The listing builds one solid part. Answer for the finished solid, in the listing's coordinates (mm). Face numbers are marked on the shaded views. A direction names the side the tool comes from. Coordinates: 2 decimals unless noted, no trailing zeros. Order: outer loops, then holes, each group sorted by start corner. A loop starts at its lowest first (then second) coordinate and runs counter-clockwise, first axis right, second up.
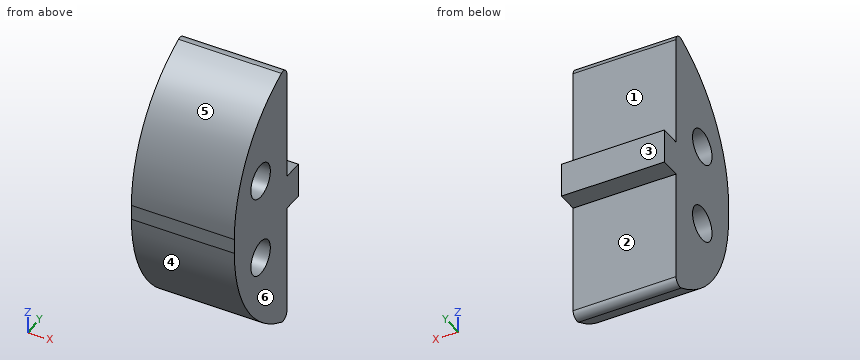
from build123d import *

# Parameters (mm, degrees)
SKETCH1_W           = 30
SKETCH1_H           = 80
BOSS_EXTRUDE1_DEPTH = 27
SKETCH5_W           = 30
SKETCH5_H           = 10
BOSS_EXTRUDE2_DEPTH = 6
SKETCH2_R           = 5
CUT_EXTRUDE1_DEPTH  = 40
FILLET5_R           = 40
FILLET6_R           = 40
FILLET7_R           = 2
FILLET8_R           = 2


with BuildPart() as part:
    # Sketch1 → Boss-Extrude1 (new body)
    with BuildSketch(Plane(origin=(0, 0, 0), x_dir=(1, 0, 0), z_dir=(0, 1, 0))):
        Rectangle(SKETCH1_W, SKETCH1_H)
    extrude(amount=BOSS_EXTRUDE1_DEPTH)

    # Sketch5 → Boss-Extrude2 (add)
    with BuildSketch(Plane(origin=(0, 27, 0), x_dir=(1, 0, 0), z_dir=(0, 1, 0))):
        Rectangle(SKETCH5_W, SKETCH5_H)
    extrude(amount=BOSS_EXTRUDE2_DEPTH)

    # Sketch2 → Cut-Extrude1 (cut)
    with BuildSketch(Plane(origin=(15, 0, 0), x_dir=(0, 0, -1), z_dir=(1, 0, 0))):
        with Locations((-12, 13.5)):
            Circle(SKETCH2_R)
        with Locations(Location((12, 13.5, 0), (0, 0, 180))):
            Circle(SKETCH2_R)
    extrude(amount=-CUT_EXTRUDE1_DEPTH, mode=Mode.SUBTRACT)

    # Fillet5
    # the kernel refuses this fillet: 40 mm, written as the material it takes off along each edge
    with BuildSketch(Plane(origin=(109.571401597, 0, -40), x_dir=(0, 0, 1), z_dir=(-1, 0, 0))) as fillet5_piece_1:
        with BuildLine():
            CenterArc((37.828560639, 40), FILLET5_R, 198.965574989, 71.034425011)
            Line((0, 27), (-0.756571213, 26.74))
            ThreePointArc((-0.756571213, 26.74), (-0.8, 13.5), (-0.8, 0))
            Line((-0.8, 0), (0, -0.8))
            Line((0, -0.8), (37.828560639, -0.8))
            Line((37.828560639, -0.8), (37.828560639, 0))
        make_face()
    extrude(amount=219.142803194, mode=Mode.SUBTRACT)

    # Fillet6
    # the kernel refuses this fillet: 40 mm, written as the material it takes off along each edge
    with BuildSketch(Plane(origin=(-109.571401597, 0, 40), x_dir=(0, 1, 0), z_dir=(1, 0, 0))) as fillet6_piece_1:
        with BuildLine():
            CenterArc((40, -37.828560639), FILLET6_R, 108.965574989, 71.034425011)
            Line((0, -37.828560639), (-0.8, -37.828560639))
            Line((-0.8, -37.828560639), (-0.8, 0))
            Line((-0.8, 0), (0, 0.8))
            ThreePointArc((0, 0.8), (13.5, 0.8), (26.74, 0.756571213))
            Line((26.74, 0.756571213), (27, 0))
        make_face()
    extrude(amount=219.142803194, mode=Mode.SUBTRACT)

    # Fillet7
    fillet7_edges = [part.edges().sort_by_distance(p)[0] for p in [
        (0, 27, -40),
    ]]
    fillet(fillet7_edges, radius=FILLET7_R)

    # Fillet8
    fillet8_edges = [part.edges().sort_by_distance(p)[0] for p in [
        (0, 27, 40),
    ]]
    fillet(fillet8_edges, radius=FILLET8_R)


solid = part.part
(1) A tool of negligible diameter and unlimited length cuts with its end or side. For the marked faces 1, 2 and 3, from which of +Z, -Z, +X, -X, +Y, -Y can it reach the whole face along a straight path? Write none if from no direction.
(2) Given pin 1 Ø15 at (x, z) = (3.5, -20.5) entering from +Y; pin 2 Ø5 at (x, y) = (2, 17.5) entering from -Z; pin 3 Ø6.5 at (x, y) = (0.5, 31.5) entering from -Z; pin 4 Ø13 at (y, z) = (13.5, -12) entering from -X, each flat-ended and moving along its own axis, determine where each tip first touches the part or whether it passes through.
(3) Find section C-C on x = -10.5. Determine the outline of the cut face in (y, z), then the cut area to 3 significant figures.
(4) Find the intervals of material crossed by probe 1 along Z at (x, y) = (-11, 10); probe 2 along Z at (x, y) = (8, 18); probe 3 along Y at (x, z) = (-2, -13.5), in increasing order.
(5) Find section D-D on z = -10. Determine the outline of the cut face in (x, y).
(6) Find section A-A on y = 14.5. Determine the outline of the cut face in (x, z).
(7) The mould has two halves that part along Z. Classify the marked faces 4, 5 and 6: pulls with the +Z half, pulls with the -Z half, needs draft (parallel to the pull), parting line crosses it, or undercut.
(8) Find section B-B on z = 12. Determine the outline of the cut face in (x, y).
Resolved:
1. face 1: +Z, +X, -X, +Y
1. face 2: -Z, +X, -X, +Y
1. face 3: +Z, -Z, +X, -X, +Y
2. pin 1: stops at y = 27
2. pin 2: stops at z = -36.81
2. pin 3: stops at z = -5
2. pin 4: stops at x = -15
3. outline: (0, -2.17) arc R40 ccw to (24.21, -38.92) arc R2 ccw to (27, -37.09) - (27, -5) - (33, -5) - (33, 5) - (27, 5) - (27, 37.09) arc R2 ccw to (24.21, 38.92) arc R40 ccw to (0, 2.17) - close; hole circle Ø10 at (13.5, -12); hole circle Ø10 at (13.5, 12)
3. area: 1,510 mm2
4. probe 1: z = -28.63 to -15.57, -8.43 to 8.43, 15.57 to 28.63
4. probe 2: z = -35.58 to -14.18, -9.82 to 9.82, 14.18 to 35.58
4. probe 3: y = 1.64 to 8.73, 18.27 to 27
5. outline: (-15, 0.77) - (15, 0.77) - (15, 8.92) - (-15, 8.92) - close; (-15, 18.08) - (15, 18.08) - (15, 27) - (-15, 27) - close
6. outline: (-15, -32.99) - (15, -32.99) - (15, -16.9) - (-15, -16.9) - close; (-15, -7.1) - (15, -7.1) - (15, 7.1) - (-15, 7.1) - close; (-15, 16.9) - (15, 16.9) - (15, 32.99) - (-15, 32.99) - close
7. face 4: pulls with the -Z half
7. face 5: pulls with the +Z half
7. face 6: needs draft
8. outline: (-15, 1.23) - (15, 1.23) - (15, 8.5) - (-15, 8.5) - close; (-15, 18.5) - (15, 18.5) - (15, 27) - (-15, 27) - close
